from build123d import *

# Parameters (mm, degrees)
IZIM1_W                          = 15
IZIM1_H                          = 30
IZIM1_R                          = 2.5
Y_KSEKLIK_EKSTR_ZYON1_DEPTH      = 5
Y_KSEKLIK_EKSTR_ZYON2_DEPTH      = 15
Y_KSEKLIK_EKSTR_ZYON2_DEPTH_BACK = 5
IZIM2_W                          = 5
IZIM2_H                          = 30
IZIM3_W                          = 15
IZIM3_H                          = 30
Y_KSEKLIK_EKSTR_ZYON3_DEPTH      = 5
IZIM4_R                          = 2.5
KES_EKSTR_ZYON1_DEPTH            = 10


with BuildPart() as part:
    # Çizim1 → Yükseklik-Ekstrüzyon1 (new body)
    with BuildSketch(Plane.XY):
        with Locations((-28.692769378, 6.725163294)):
            Rectangle(IZIM1_W, IZIM1_H)
        with Locations((-31.192769378, 14.225163294)):
            Circle(IZIM1_R, mode=Mode.SUBTRACT)
        with Locations((-31.192769378, -0.774836706)):
            Circle(IZIM1_R, mode=Mode.SUBTRACT)
    extrude(amount=Y_KSEKLIK_EKSTR_ZYON1_DEPTH)

    # Çizim2 → Yükseklik-Ekstrüzyon2 (add, two sides: drawn at the far end of the back side and taken through both)
    with BuildSketch(Plane(origin=(0, 0, 0), x_dir=(-1, 0, 0), z_dir=(0, 0, -1)).offset(-Y_KSEKLIK_EKSTR_ZYON2_DEPTH_BACK)):
        with Locations((38.692769378, 6.725163294)):
            Rectangle(IZIM2_W, IZIM2_H)
    extrude(amount=Y_KSEKLIK_EKSTR_ZYON2_DEPTH + Y_KSEKLIK_EKSTR_ZYON2_DEPTH_BACK)

    # Çizim3 → Yükseklik-Ekstrüzyon3 (add)
    with BuildSketch(Plane(origin=(0, 0, -15), x_dir=(-1, 0, 0), z_dir=(0, 0, -1))):
        with Locations((48.692769378, 6.725163294)):
            Rectangle(IZIM3_W, IZIM3_H)
    extrude(amount=-Y_KSEKLIK_EKSTR_ZYON3_DEPTH)

    # Çizim4 → Kes-Ekstrüzyon1 (cut)
    with BuildSketch(Plane.XY.offset(-10)):
        with Locations((-46.192769378, 14.225163294)):
            Circle(IZIM4_R)
        with Locations((-46.192769378, -0.774836706)):
            Circle(IZIM4_R)
    extrude(amount=-KES_EKSTR_ZYON1_DEPTH, mode=Mode.SUBTRACT)


solid = part.part
Verification items for the finished model (mm, model axes). A direction names the side the tool comes from. Round coordinates to 2 decimals unless told otherwise and drop trailing zeros. Loops run counter-clockwise (first coordinate to the right, second up) from the corner with the lowest first, then second, coordinate; pieces in that order, holes last. Notation, with made-up numbers: M 86.5,4 L 125.5,4 A22 ccw 125.5,34 Z; hole C 58,55.25 d8. An arc over 180 degrees is marked long. Write each question's results on one line, items separated by ' | '.
1) Mould release check, pull along X, two halves, no side actions. Record for faces 1 (the flat face through (-36.193, 7, -7)), 2 (the cylindrical face through (-28.883, 13.268, 2.465)), 3 (the flat face through (-39, 21.725, -6)): released by +X, released by -X, zero draft, split by the parting line, or undercut.
Checks:
face 1: released by +X | face 2: undercut | face 3: zero draft
2) Section check B-B on x = -31.5. Record the boundary of the cut face in (y, z).
Checks:
outline: M -8.27,0 L -3.26,0 L -3.26,5 L -8.27,5 Z; M 1.71,0 L 11.74,0 L 11.74,5 L 1.71,5 Z; M 16.71,0 L 21.73,0 L 21.73,5 L 16.71,5 Z
3) Section check D-D on z = 1. Record the boundary of the cut face in (x, y), then the cut area to 3 significant figures.
Checks:
outline: M -41.19,-8.27 L -21.19,-8.27 L -21.19,21.73 L -41.19,21.73 Z; hole C -31.19,-0.77 d5; hole C -31.19,14.23 d5 | area: 561 mm2
4) Section check C-C on y = -2.75. Record the boundary of the cut face in (x, z).
Checks:
outline: M -56.19,-15 L -47.73,-15 L -47.73,-10 L -56.19,-10 Z; M -44.66,-15 L -36.19,-15 L -36.19,0 L -32.73,0 L -32.73,5 L -41.19,5 L -41.19,-10 L -44.66,-10 Z; M -29.66,0 L -21.19,0 L -21.19,5 L -29.66,5 Z
5) Scan lines: L1, parallel to Y at x = -47, z = -10.5; L2, parallel to X at y = 19.5, z = -9.5; L3, parallel to X at y = 3, z = 4. Record each from-to range of solid material in increasing order. Write a range as from..to.
Checks:
L1: y = -8.27..-3.14, 1.59..11.86, 16.59..21.73 | L2: x = -41.19..-36.19 | L3: x = -41.19..-21.19
6) Gauge pin test, flat ends, axial feed: P1, Ø8, axis at x = -46.19, y = -0.77, coming from the -Z side; P2, Ø12, axis at x = -26, y = 13.5, coming from the -Z side; P3, Ø4.5, axis at x = -51, y = 9.5, coming from the +Z side; P4, Ø2, axis at x = -43.5, z = -8.5, coming from the +Y side. Record the tip position at first contact, or that the pin passes through.
Checks:
P1: stops at z = -15 | P2: stops at z = 0 | P3: stops at z = -10 | P4: passes through
7) Section check A-A on y = 5.25. Record the boundary of the cut face in (x, z).
Checks:
outline: M -56.19,-15 L -36.19,-15 L -36.19,0 L -21.19,0 L -21.19,5 L -41.19,5 L -41.19,-10 L -56.19,-10 Z
8) Access from +Z, -Z, +X, -X, +Y, -Y to the whole of each face (thin tool, end or side, straight path). Record for faces 4 (the flat face through (-29, 7, 0)), 5 (the flat face through (-46, 7, -15)), 6 (the flat face through (-49, 7, -10)).
Checks:
face 4: -Z, +X, +Y, -Y | face 5: -Z, +X, -X, +Y, -Y | face 6: +Z, -X, +Y, -Y
